from build123d import *

# Parameters (mm, degrees)
BRIDA_START                  = 567
SK_BRIDA_R                   = 31.5
BRIDA_DEPTH                  = 8
CENTRO_START                 = 567
SK_CENTRO_R                  = 3
CENTRO_DEPTH                 = 8
ROSCAS_M4_HERRAMIENTA_START  = 567
SK_ROSCAS_M4_HERRAMIENTA_R   = 1.65
ROSCAS_M4_HERRAMIENTA_DEPTH  = 8
PASANTES_M2_5_ROTOR_J6_START = 567
SK_PASANTES_M2_5_ROTOR_J6_R  = 1.45
PASANTES_M2_5_ROTOR_J6_DEPTH = 8
CAJAS_M2_5_START             = 572.5
SK_CAJAS_M2_5_R              = 2.75
CAJAS_M2_5_DEPTH             = 2.5


with BuildPart() as part:
    # Sk_Brida → Brida (new body)
    with BuildSketch(Plane.XY.offset(BRIDA_START)):
        Circle(SK_BRIDA_R)
    extrude(amount=BRIDA_DEPTH)

    # Sk_Centro → Centro (cut)
    with BuildSketch(Plane.XY.offset(CENTRO_START)):
        Circle(SK_CENTRO_R)
    extrude(amount=CENTRO_DEPTH, mode=Mode.SUBTRACT)

    # Sk_Roscas_M4_herramienta → Roscas_M4_herramienta (cut)
    with BuildSketch(Plane.XY.offset(ROSCAS_M4_HERRAMIENTA_START)):
        with Locations((14.142135624, 14.142135624)):
            Circle(SK_ROSCAS_M4_HERRAMIENTA_R)
        with Locations((-14.142135624, 14.142135624)):
            Circle(SK_ROSCAS_M4_HERRAMIENTA_R)
        with Locations((-14.142135624, -14.142135624)):
            Circle(SK_ROSCAS_M4_HERRAMIENTA_R)
        with Locations((14.142135624, -14.142135624)):
            Circle(SK_ROSCAS_M4_HERRAMIENTA_R)
    extrude(amount=ROSCAS_M4_HERRAMIENTA_DEPTH, mode=Mode.SUBTRACT)

    # Sk_Pasantes_M2-5_rotor_J6 → Pasantes_M2-5_rotor_J6 (cut)
    with BuildSketch(Plane.XY.offset(PASANTES_M2_5_ROTOR_J6_START)):
        with Locations((12.390194253, -1.653204878)):
            Circle(SK_PASANTES_M2_5_ROTOR_J6_R)
        with Locations((7.626814549, 9.903620542)):
            Circle(SK_PASANTES_M2_5_ROTOR_J6_R)
        with Locations((-4.763379704, 11.55682542)):
            Circle(SK_PASANTES_M2_5_ROTOR_J6_R)
        with Locations((-12.390194253, 1.653204878)):
            Circle(SK_PASANTES_M2_5_ROTOR_J6_R)
        with Locations((-7.626814549, -9.903620542)):
            Circle(SK_PASANTES_M2_5_ROTOR_J6_R)
        with Locations((4.763379704, -11.55682542)):
            Circle(SK_PASANTES_M2_5_ROTOR_J6_R)
    extrude(amount=PASANTES_M2_5_ROTOR_J6_DEPTH, mode=Mode.SUBTRACT)

    # Sk_Cajas_M2-5 → Cajas_M2-5 (cut)
    with BuildSketch(Plane.XY.offset(CAJAS_M2_5_START)):
        with Locations((12.390194253, -1.653204878)):
            Circle(SK_CAJAS_M2_5_R)
        with Locations((7.626814549, 9.903620542)):
            Circle(SK_CAJAS_M2_5_R)
        with Locations((-4.763379704, 11.55682542)):
            Circle(SK_CAJAS_M2_5_R)
        with Locations((-12.390194253, 1.653204878)):
            Circle(SK_CAJAS_M2_5_R)
        with Locations((-7.626814549, -9.903620542)):
            Circle(SK_CAJAS_M2_5_R)
        with Locations((4.763379704, -11.55682542)):
            Circle(SK_CAJAS_M2_5_R)
    extrude(amount=CAJAS_M2_5_DEPTH, mode=Mode.SUBTRACT)


solid = part.part
Source: CAD feature listing. Evaluate the final solid. Frame: model axes, mm. A direction names the side the tool comes from. Round coordinates to 2 decimals unless told otherwise and drop trailing zeros. Write each loop counter-clockwise with the first axis right and the second up, starting at its lowest first coordinate (ties: lowest second). Pieces come first, ordered by that corner, then holes. Notation, with made-up numbers: (16.25, 89.5) - (53.25, 89.5) arc R31 cw to (53.25, 122.5) - close; hole circle Ø4 at (-7.5, 42.25). An arc over 180 degrees is marked (long way). Use CSV: the item, a comma, the result in double quotes. Start each with the question number.
(1) Mould query, pull axis X, two halves, no side actions, for faces 3 (the face through (6.146, -11.121, 569.712)), 4 (the face through (7, 0, 567)), 5 (the face through (-11, 0, 572.5)). Classes: pulls with the +X half, pulls with the -X half, needs draft (parallel to the pull), parting line crosses it, or undercut.
(2) Material intervals for probe 1 along Y at (x, z) = (14, 568); probe 2 along X at (y, z) = (-2, 574); probe 3 along X at (y, z) = (11, 569), sorted ascending. Write a range as [from, to].
(3) Cut plane B-B, the plane z = 574.25. Give the number of separate pieces and of enclosed holes in the cut face, and give its area (3 significant figures).
(4) Set-up query: faces 1 (the face through (-6.244, -9.468, 569.712)), 2 (the face through (-6, -11, 572.5)). Return all of +Z, -Z, +X, -X, +Y, -Y with unobstructed straight access to the full face (end or side cutting, diameter ignored); none if empty.
(5) Cut plane A-A, the plane x = 0. Return loops of the section in (y, z), and give its area (3 significant figures).
(6) First-contact query: pin 1 Ø1.7 at (x, y) = (4.76, -11.56) entering from -Z; pin 2 Ø6.5 at (x, y) = (4.76, -11.56) entering from -Z; pin 3 Ø1.6 at (x, y) = (-7, -10.5) entering from +Z; pin 4 Ø3 at (y, z) = (22.5, 573) entering from +X. Flat tips, straight axial feed; report the tip coordinate or a pass-through.
(7) Cut plane D-D, the plane y = 19. Return loops of the section in (x, z).
Geometry says:
1,face 3,"undercut"
1,face 4,"needs draft"
1,face 5,"undercut"
2,probe 1,"[-28.22, -15.79], [-12.5, 12.5], [15.79, 28.22]"
2,probe 2,"[-31.44, -2.24], [2.24, 9.66], [15.12, 31.44]"
2,probe 3,"[-29.52, -6.1], [-3.42, 6.68], [8.58, 29.52]"
3,separate pieces,"1"
3,enclosed holes,"11"
3,area,"2,910 mm²"
4,face 1,"+Z, -Z"
4,face 2,"+Z"
5,outline,"(-31.5, 567) - (-3, 567) - (-3, 575) - (-31.5, 575) - close; (3, 567) - (31.5, 567) - (31.5, 575) - (3, 575) - close"
5,area,"456 mm²"
6,pin 1,"through"
6,pin 2,"z = 567"
6,pin 3,"z = 572.5"
6,pin 4,"x = 23.48"
7,outline,"(-25.12, 567) - (25.12, 567) - (25.12, 575) - (-25.12, 575) - close"
